Here's how the part is built. I have some questions about the finished solid (model axes, mm). A direction names the side the tool comes from. Round coordinates to 2 decimals unless told otherwise and drop trailing zeros. Loops run counter-clockwise (first coordinate to the right, second up) from the corner with the lowest first, then second, coordinate; pieces in that order, holes last. Notation, with made-up numbers: (-39.5, 1.5) - (-8.5, 1.5) arc R32 cw to (-8.5, 38.5) - close; hole circle Ø8 at (44, -24). An arc over 180 degrees is marked (long way). Answer as a JSON object with one key per item and string values. Group by question number.
1) I want a section at A-A, the plane x = 0.95. Please give me the cut outline in (y, z), then the cut area to 3 significant figures.
2) I want a section at B-B, the plane z = 0. Please give me the cut outline in (x, y), then the cut area to 3 significant figures.
3) If I drill on line 1 along X through (y, z) = (0.6, 0); line 2 along Y through (x, z) = (0.3, 1.65); line 3 along Y through (x, z) = (1.7, -1.2), over which ranges is the centre line in solid material (lowest first)? Write a range as [from, to].
4) I want a section at C-C, the plane x = 0. Please give me the cut outline in (y, z), then the cut area to 3 significant figures.
5) If we mould it in two halves opening along X, with no side actions, what happens to faces 1 (the face through (0, 3.113, 1)), 2 (the face through (0.1, 1, -2.9)), 3 (the face through (-1.952, 0.493, 0.434))? For each: pulls with the +X half, pulls with the -X half, needs draft (parallel to the pull), parting line crosses it, or undercut.
6) Will these pins go through, and if not, where does the flat tip stop? P1, Ø1, axis at x = 0, y = 3, coming from the -Z side; P2, Ø3, axis at x = 0.5, z = 1, coming from the -Y side.
7) Which directions (+Z, -Z, +X, -X, +Y, -Y) give clear straight access to the entire face, cutting with the end or side of a thin tool? Please do faces 4 (the face through (0, 1, 0)), 5 (the face through (-2, 0, -1)), 6 (the face through (-0.119, 2.549, 0.534)), 7 (the face through (-2.043, 3.576, -1.873)), 8 (the face through (0, 4.052, 0)).
8) I want a section at D-D, the plane z = -1. Please give me the cut outline in (x, y), then the cut area to 3 significant figures.
from build123d import *

# Parameters (mm, degrees)
SKETCH1_R           = 2.9
BOSS_EXTRUDE1_DEPTH = 2
SKETCH2_R           = 2
CUT_EXTRUDE1_DEPTH  = 1


with BuildPart() as part:
    # Sketch1 → Boss-Extrude1 (new body)
    with BuildSketch(Plane(origin=(0, 0, 0), x_dir=(1, 0, 0), z_dir=(0, 1, 0))):
        with Locations(Location((0, 0, 0), (0, 0, 270))):
            Circle(SKETCH1_R)
    extrude(amount=BOSS_EXTRUDE1_DEPTH)

    # Sketch2 → Cut-Extrude1 (cut)
    with BuildSketch(Plane.XZ):
        with Locations(Location((0, 0, 0), (0, 0, 270))):
            Circle(SKETCH2_R)
    extrude(amount=-CUT_EXTRUDE1_DEPTH, mode=Mode.SUBTRACT)

    # Sketch3 → Revolve4 (revolve)
    with BuildSketch(Plane.XY, mode=Mode.PRIVATE) as revolve4_sk:
        Polygon((-2.771365676, 3.112953388), (-0.547366303, 3.112953388), (-0.547366303, 2), (0, 2), (0, 4.051740853), (-2.771365676, 4.051740853), align=None)
    revolve(revolve4_sk.sketch.rotate(Axis((0, 2, 0), (0, 1, 0)), 180), axis=Axis((0, 2, 0), (0, 1, 0)))


solid = part.part
Outcome:
{
 "1": {"outline": "(0, -2.74) - (2, -2.74) - (2, 2.74) - (0, 2.74) - (0, 1.76) - (1, 1.76) - (1, -1.76) - (0, -1.76) - close; (3.11, -2.6) - (4.05, -2.6) - (4.05, 2.6) - (3.11, 2.6) - close", "area": "12.3 mm^2"},
 "2": {"outline": "(-2.9, 0) - (-2, 0) - (-2, 1) - (2, 1) - (2, 0) - (2.9, 0) - (2.9, 2) - (0.55, 2) - (0.55, 3.11) - (2.77, 3.11) - (2.77, 4.05) - (-2.77, 4.05) - (-2.77, 3.11) - (-0.55, 3.11) - (-0.55, 2) - (-2.9, 2) - close", "area": "14.0 mm^2"},
 "3": {"line 1": "[-2.9, -2], [2, 2.9]", "line 2": "[1, 2], [3.11, 4.05]", "line 3": "[0, 2], [3.11, 4.05]"},
 "4": {"outline": "(0, -2.9) - (2, -2.9) - (2, -0.55) - (3.11, -0.55) - (3.11, -2.77) - (4.05, -2.77) - (4.05, 2.77) - (3.11, 2.77) - (3.11, 0.55) - (2, 0.55) - (2, 2.9) - (0, 2.9) - (0, 2) - (1, 2) - (1, -2) - (0, -2) - close", "area": "14.0 mm^2"},
 "5": {"face 1": "needs draft", "face 2": "parting line crosses it", "face 3": "undercut"},
 "6": {"P1": "z = -2.77", "P2": "y = 0"},
 "7": {"face 4": "-Y", "face 5": "+Z, -Z, +X, -X, -Y", "face 6": "none", "face 7": "+Y", "face 8": "+Z, -Z, +X, -X, +Y"},
 "8": {"outline": "(-2.72, 0) - (-1.73, 0) - (-1.73, 1) - (1.73, 1) - (1.73, 0) - (2.72, 0) - (2.72, 2) - (-2.72, 2) - close; (-2.58, 3.11) - (2.58, 3.11) - (2.58, 4.05) - (-2.58, 4.05) - close", "area": "12.3 mm^2"}
}
